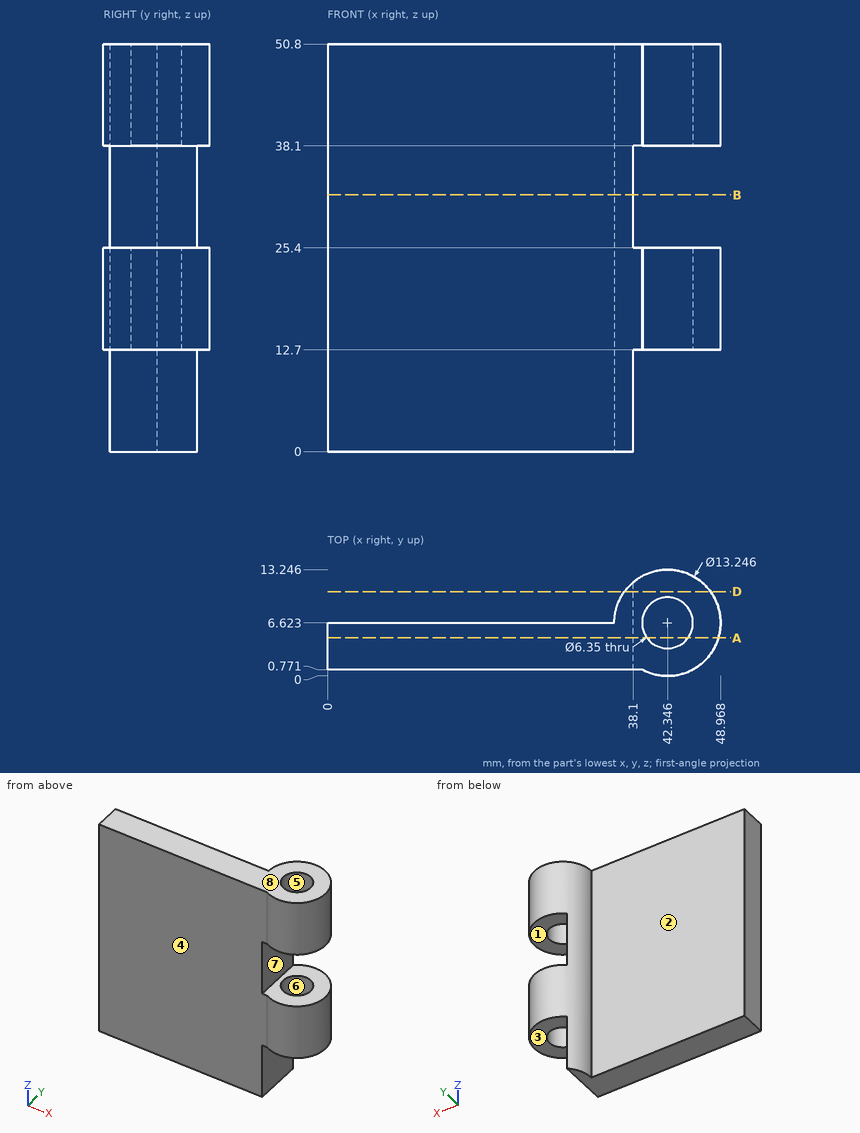
Geometry check sheet. Reference: drawing and pictorial views, mm from the part's lowest x, y, z. A direction names the side the tool comes from. Round coordinates to 2 decimals unless told otherwise and drop trailing zeros. Loops run counter-clockwise (first coordinate to the right, second up) from the corner with the lowest first, then second, coordinate; pieces in that order, holes last. Notation, with made-up numbers: (51, 66.5) -> (99, 66.5) arc R14 ccw to (99, 74.5) -> close; hole circle Ø2 at (-39.75, 58.5). An arc over 180 degrees is marked (long way). Answer as a JSON object with one key per item and string values.
Q1. Draft check along X on the marked faces 5, 6, 7 and 8. Enter one of: pulls with the +X half, pulls with the -X half, needs draft (parallel to the pull), parting line crosses it, or undercut.
Data:
{"face 5": "undercut", "face 6": "undercut", "face 7": "pulls with the +X half", "face 8": "needs draft"}
Q2. Section check A-A (y = 4.75). Record the boundary of the cut face in (x, z).
Data:
{"outline": "(0, 0) -> (38.1, 0) -> (38.1, 12.7) -> (39.78, 12.7) -> (39.78, 25.4) -> (38.1, 25.4) -> (38.1, 38.1) -> (39.78, 38.1) -> (39.78, 50.8) -> (0, 50.8) -> close; (44.91, 12.7) -> (48.7, 12.7) -> (48.7, 25.4) -> (44.91, 25.4) -> close; (44.91, 38.1) -> (48.7, 38.1) -> (48.7, 50.8) -> (44.91, 50.8) -> close"}
Q3. Section check D-D (y = 10.5). Record the boundary of the cut face in (x, z) (1 decimal), then the cut area to 3 significant figures.
Data:
{"outline": "(37, 0) -> (38.1, 0) -> (38.1, 12.7) -> (47.7, 12.7) -> (47.7, 25.4) -> (38.1, 25.4) -> (38.1, 38.1) -> (47.7, 38.1) -> (47.7, 50.8) -> (37, 50.8) -> close", "area": "301 mm2"}
Q4. Access from +Z, -Z, +X, -X, +Y, -Y to the whole of each face (thin tool, end or side, straight path). Record for the marked faces 1, 2, 3 and 4.
Data:
{"face 1": "+X, +Y, -Y", "face 2": "+Z, -Z, -X, +Y", "face 3": "-Z, +X, +Y, -Y", "face 4": "+Z, -Z, -X, -Y"}
Q5. Section check B-B (z = 32). Record the boundary of the cut face in (x, y) (1 decimal), then the cut area to 3 significant figures.
Data:
{"outline": "(0, 0.8) -> (38.1, 0.8) -> (38.1, 11.7) arc R6.6 ccw to (35.7, 6.6) -> (0, 6.6) -> close", "area": "231 mm2"}
Q6. Go/stop test with flat-tipped pins: P1, Ø2, axis at x = 5, z = 44.5, coming from the -Y side; P2, Ø5.5, axis at x = 42.35, y = 6.62, coming from the +Z side; P3, Ø7.5, axis at x = 42.35, y = 6.62, coming from the -Z side; P4, Ø4, axis at x = 10.5, z = 30.5, coming from the +Y side. Record where each tip stops, or that it passes through.
Data:
{"P1": "stops at y = 0.77", "P2": "passes through", "P3": "stops at z = 12.7", "P4": "stops at y = 6.62"}
Q7. Scan lines: line 1 (Z direction, x = 42, y = 2.25); line 2 (X direction, y = 2, z = 30); line 3 (Y direction, x = 21.5, z = 27). Record each from-to range of solid material in increasing order. Write a range as from..to.
Data:
{"line 1": "z = 12.7..25.4, 38.1..50.8", "line 2": "x = 0..38.1", "line 3": "y = 0.77..6.62"}
